from build123d import *

# Parameters (mm, degrees)
F0_W         = 110
F0_H         = 30
F1_DEPTH     = 2
F3_DEPTH     = 55
F5_DEPTH     = 2.3635386072
F7_DEPTH     = 2
F9_DEPTH     = 1
F10_W        = 43
F10_H        = 15.6
F11_DEPTH    = 2
F12_T1_DEPTH = 27.4
F13_R        = 4


# Not quite as in the source:
# - a fillet or chamfer that OpenCascade refuses, or shapes differently, is made with other operations: its cross-section is extruded or revolved along the edge and cut away or added
# - a pattern or mirror of a feature is missing from the dataset's text; its kind, count and spacing are read off the source's solid


with BuildPart() as f1:
    # F0 (on Top) → F1 (new body)
    with BuildSketch(Plane.XY):
        Rectangle(F0_W, F0_H)
    extrude(amount=F1_DEPTH)

    # F2 (on Right) → F3 (join, symmetric)
    with BuildSketch(Plane.YZ):
        Polygon((-15, 2), (-12.6, 2), (-5.5469207717, 42), (-7.9469207717, 42), align=None)
    extrude(amount=F3_DEPTH, both=True)

    # F4 (on face) → F5 (cut, through all)
    with BuildSketch(Plane(origin=(0, -14.8897147992, 2.6254584542), x_dir=(1, 0, 0), z_dir=(0, -0.984807753, 0.1736481777))):
        with BuildLine():
            Line((-9, 21.9819573165), (-9, 39.9819573165))
            Line((-9, 39.9819573165), (-9, 44.9819573165))
            Line((-9, 44.9819573165), (-45, 44.9819573165))
            Line((-45, 44.9819573165), (-45, 39.9819573165))
            Line((-45, 39.9819573165), (-45, 21.9819573165))
            ThreePointArc((-45, 21.9819573165), (-27, 3.9819573165), (-9, 21.9819573165))
        make_face()
    f5 = extrude(amount=-F5_DEPTH, mode=Mode.SUBTRACT)

    # F5_copies: F5 across plane
    add(f5.mirror(Plane(origin=(0, 0, 0), x_dir=(0, 0, 1), z_dir=(1, 0, 0))), mode=Mode.SUBTRACT)

    # F6 (on face) → F7 (join)
    with BuildSketch(Plane(origin=(-55, 0, 0), x_dir=(0, -1, 0), z_dir=(-1, 0, 0))):
        Polygon((7.39055467, 31.5442325904), (-7.4, 2), (12.6, 2), align=None)
    f7 = extrude(amount=-F7_DEPTH)

    # F7_copies: F7 across plane
    add(f7.mirror(Plane(origin=(0, 0, 0), x_dir=(0, 0, 1), z_dir=(1, 0, 0))))

    # F8 (on Right) → F9 (join, symmetric)
    with BuildSketch(Plane.YZ):
        Polygon((-12.6, 2), (7.4, 2), (-7.39055467, 31.5442325904), align=None)
    extrude(amount=F9_DEPTH, both=True)

    # F10 (on Top) → F11 (cut, through all)
    with BuildSketch(Plane.XY):
        with Locations((27.5, 1.2)):
            Rectangle(F10_W, F10_H)
        with Locations((-27.5, 1.2)):
            Rectangle(F10_W, F10_H)
    extrude(amount=F11_DEPTH, mode=Mode.SUBTRACT)

    # F12: fillet of radius 5 on 6 edges, made by hand

    # F12_s2 → F12_t1 (cut)
    with BuildSketch(Plane.XZ.offset(-6.9530792283)):
        with BuildLine():
            ThreePointArc((50, 42), (46.4644660941, 40.5355339059), (45, 37))
            Line((45, 37), (45, 42))
            Line((45, 42), (50, 42))
        make_face()
        with BuildLine():
            ThreePointArc((-45, 37), (-46.4644660941, 40.5355339059), (-50, 42))
            Line((-50, 42), (-45, 42))
            Line((-45, 42), (-45, 37))
        make_face()
        with BuildLine():
            ThreePointArc((-9, 37), (-7.5355339059, 40.5355339059), (-4, 42))
            Line((-4, 42), (-9, 42))
            Line((-9, 42), (-9, 37))
        make_face()
        with BuildLine():
            ThreePointArc((4, 42), (7.5355339059, 40.5355339059), (9, 37))
            Line((9, 37), (9, 42))
            Line((9, 42), (4, 42))
        make_face()
    extrude(amount=F12_T1_DEPTH, mode=Mode.SUBTRACT)

    # F13
    f13_edges = [f1.edges().sort_by_distance(p)[0] for p in [
        (-49, -6.6, 1),
        (49, -6.6, 1),
        (-6, -6.6, 1),
        (6, -6.6, 1),
        (6, 9, 1),
        (-49, 9, 1),
        (49, 9, 1),
        (-6, 9, 1),
    ]]
    fillet(f13_edges, radius=F13_R)


solid = f1.part
CAD build for the part. Positions are in the model's coordinates, mm. A direction names the side the tool comes from. Round coordinates to 2 decimals unless told otherwise and drop trailing zeros. Loops run counter-clockwise (first coordinate to the right, second up) from the corner with the lowest first, then second, coordinate; pieces in that order, holes last.
(1) Two-plate mould, pull along X, no slides. Class faces 6 (the cylindrical face through (-47.797, 7.859, 1.014)), 7 (the flat face through (-1, 15, 1)), 8 (the flat face through (-55, -5, 13)): +X half, -X half, draft (parallel to the pull), parting line (faces both ways), or undercut.
(2) Wall check: line 1 along X through (y, z) = (-7, 20); line 2 along X through (y, z) = (-11.5, 19.5); line 3 along Z through (x, y) = (-15, 10.5). Give the ranges that are in metal, low to high.
(3) Cut at D-D (z = 5). Give the cut face in (x, y).
(4) Drop flat-ended pins along their axis: pin 1 (2 mm diameter, centred on x = 16.5, y = 12, fed in from +Z); pin 2 (4 mm diameter, centred on x = -14, y = -5.5, fed in from -Z). Give the stop position or say it passes through.
(5) Cut at B-B (x = 25). Give the cut face in (y, z).
(6) Cut at A-A (z = 38.5). Give the cut face in (x, y), plus the area to 3 significant figures.
(7) Which spindle directions (+Z, -Z, +X, -X, +Y, -Y) get a long thin tool onto all of the face, cutting with end or side? Do faces 1 (the cylindrical face through (7.203, 7.859, 1.014)), 2 (the flat face through (-9, -9, 31)), 3 (the flat face through (-1, 8, 2)), 4 (the cylindrical face through (7.203, -5.459, 1.014)), 5 (the flat face through (-1, 0, 0)). Say none if no direction does.
(8) Cut at C-C (y = 6.25). Give the cut face in (x, z), plus the area to 3 significant figures.
Findings below:
1. face 6: undercut
1. face 7: draft
1. face 8: -X half
2. line 1: x = -55 to -53, -1 to 1, 53 to 55
2. line 2: x = -55 to -44.36, -9.64 to 9.64, 44.36 to 55
2. line 3: z = 0 to 2
3. outline: (-55, -14.47) - (55, -14.47) - (55, 5.9) - (53, 5.9) - (53, -12.07) - (1, -12.07) - (1, 5.9) - (-1, 5.9) - (-1, -12.07) - (-53, -12.07) - (-53, 5.9) - (-55, 5.9) - close
4. pin 1: stops at z = 2
4. pin 2: stops at z = 0
5. outline: (-15, 0) - (-6.6, 0) - (-6.6, 2) - (-12.6, 2) - (-11.85, 6.25) - (-14.18, 6.66) - (-15, 2) - close; (9, 0) - (15, 0) - (15, 2) - (9, 2) - close
6. outline: (-55, -8.56) - (-45.23, -8.56) - (-45.23, -6.16) - (-55, -6.16) - close; (-8.77, -8.56) - (8.77, -8.56) - (8.77, -6.16) - (-8.77, -6.16) - close; (45.23, -8.56) - (55, -8.56) - (55, -6.16) - (45.23, -6.16) - close
6. area: 89.0 mm2
7. face 1: +Z, -Z
7. face 2: +Z, +Y, -Y
7. face 3: +Y
7. face 4: -Z
7. face 5: -Z, +X, -X, +Y, -Y
8. outline: (-55, 0) - (-48.8, 0) - (-48.8, 2) - (-53, 2) - (-53, 4.3) - (-55, 4.3) - close; (-6.2, 0) - (6.2, 0) - (6.2, 2) - (1, 2) - (1, 4.3) - (-1, 4.3) - (-1, 2) - (-6.2, 2) - close; (48.8, 0) - (55, 0) - (55, 4.3) - (53, 4.3) - (53, 2) - (48.8, 2) - close
8. area: 63.4 mm2
